Source: CAD feature listing. Evaluate the final solid. Frame: model axes, mm. A direction names the side the tool comes from. Coordinates: 2 decimals unless noted, no trailing zeros. Write each loop counter-clockwise with the first axis right and the second up, starting at its lowest first coordinate (ties: lowest second). Pieces come first, ordered by that corner, then holes. Notation, with made-up numbers: (-7.5, 42) - (50.5, 42) arc R7 cw to (50.5, 54) - close; hole circle Ø10 at (55, -12). An arc over 180 degrees is marked (long way). One line per item, written item: value.
from build123d import *

# Parameters (mm, degrees)
CROQUIS1_W              = 5.5
CROQUIS1_H              = 7
CROQUIS1_W_2            = 5
CROQUIS1_H_2            = 3
SALIENTE_EXTRUIR1_DEPTH = 20
CROQUIS2_W              = 5.5
CROQUIS2_H              = 7
CORTAR_EXTRUIR3_DEPTH   = 37.932370625
CROQUIS3_R              = 1.5
CORTAR_EXTRUIR4_DEPTH   = 33.015621187
REDONDEO1_R             = 3
CROQUIS4_R              = 1.5
CORTAR_EXTRUIR5_DEPTH   = 31.724582991
SALIENTE_EXTRUIR2_DEPTH = 20
CROQUIS9_R              = 2.75
CORTAR_EXTRUIR6_DEPTH   = 2.5


with BuildPart() as part:
    # Croquis1 → Saliente-Extruir1 (new body)
    with BuildSketch(Plane.XY):
        with Locations((-7.25, 3.5)):
            Rectangle(CROQUIS1_W, CROQUIS1_H)
        Polygon((0, -5), (0, -8), (-10, 0), (-4.5, 0), align=None)
        with Locations((2.5, -6.5)):
            Rectangle(CROQUIS1_W_2, CROQUIS1_H_2)
        with Locations((7.5, -6.5)):
            Rectangle(CROQUIS1_W_2, CROQUIS1_H_2)
        Polygon((14.5, 0), (20, 0), (10, -8), (10, -5), align=None)
        with Locations((17.25, 3.5)):
            Rectangle(CROQUIS1_W, CROQUIS1_H)
    extrude(amount=SALIENTE_EXTRUIR1_DEPTH)

    # Croquis2 → Cortar-Extruir3 (cut, through all)
    with BuildSketch(Plane.ZY.offset(10)):
        with Locations((15, 0)):
            Rectangle(CROQUIS2_W, CROQUIS2_H)
        with Locations((5, 0)):
            Rectangle(CROQUIS2_W, CROQUIS2_H)
    extrude(amount=-CORTAR_EXTRUIR3_DEPTH, mode=Mode.SUBTRACT)

    # Croquis3 → Cortar-Extruir4 (cut, through all)
    with BuildSketch(Plane(origin=(0, 7, 0), x_dir=(1, 0, 0), z_dir=(0, 1, 0))):
        with Locations(Location((-7.25, -5, 0), (0, 0, 180))):
            Circle(CROQUIS3_R)
        with Locations(Location((17.75, -5, 0), (0, 0, 180))):
            Circle(CROQUIS3_R)
        with Locations(Location((17.75, -15, 0), (0, 0, 180))):
            Circle(CROQUIS3_R)
        with Locations(Location((-7.25, -15, 0), (0, 0, 180))):
            Circle(CROQUIS3_R)
    extrude(amount=-CORTAR_EXTRUIR4_DEPTH, mode=Mode.SUBTRACT)

    # Redondeo1
    redondeo1_edges = [part.edges().sort_by_distance(p)[0] for p in [
        (20, 0, 18.875),
        (10, -8, 10),
        (0, -8, 10),
        (-10, 0, 18.875),
        (20, 0, 10),
        (20, 0, 1.125),
        (-10, 0, 10),
        (-10, 0, 1.125),
    ]]
    fillet(redondeo1_edges, radius=REDONDEO1_R)

    # Croquis4 → Cortar-Extruir5 (cut, through all)
    with BuildSketch(Plane(origin=(0, -5, 0), x_dir=(1, 0, 0), z_dir=(0, 1, 0))):
        with Locations(Location((5, -10, 0), (0, 0, 180))):
            Circle(CROQUIS4_R)
    extrude(amount=-CORTAR_EXTRUIR5_DEPTH, mode=Mode.SUBTRACT)

    # Croquis8 → Saliente-Extruir2 (add, through all)
    with BuildSketch(Plane(origin=(0, 0, 0), x_dir=(-1, 0, 0), z_dir=(0, 0, -1))):
        Polygon((-5, -5), (0, -5), (1.29685781, -3.559046878), (-5, -3.559046878), align=None)
        Polygon((-10, -5), (-5, -5), (-5, -3.559046878), (-11.29685781, -3.559046878), align=None)
    extrude(amount=-SALIENTE_EXTRUIR2_DEPTH)

    # Croquis9 → Cortar-Extruir6 (cut)
    with BuildSketch(Plane(origin=(0, -3.559046878, 0), x_dir=(1, 0, 0), z_dir=(0, 1, 0))):
        with Locations(Location((5, -10, 0), (0, 0, 180))):
            Circle(CROQUIS9_R)
    extrude(amount=-CORTAR_EXTRUIR6_DEPTH, mode=Mode.SUBTRACT)


solid = part.part
1) Section query C-C on z = 10. Output: boundary loops of the cut face in (x, y).
Values found:
outline: (-10, 1.44) arc R3 ccw to (-8.87, -0.9) - (-0.82, -7.34) arc R3 ccw to (1.05, -8) - (3.5, -8) - (3.5, -6.06) - (2.25, -6.06) - (2.25, -3.56) - (-1.3, -3.56) - (-4.5, 0) - (-4.5, 7) - (-10, 7) - close; (6.5, -8) - (8.95, -8) arc R3 ccw to (10.82, -7.34) - (18.87, -0.9) arc R3 ccw to (20, 1.44) - (20, 7) - (14.5, 7) - (14.5, 0) - (11.3, -3.56) - (7.75, -3.56) - (7.75, -6.06) - (6.5, -6.06) - close
2) Reachability of faces 4 (the flat face through (3.8, -6.059, 8.8)), 5 (the flat face through (2, -3.559, 10)), 6 (the flat face through (-7, 0, 2.25)), 7 (the cylindrical face through (-9.712, 0.159, 10.032)) from +Z, -Z, +X, -X, +Y, -Y: full face, straight path, thin tool, end or side. Return the list, or none.
Values found:
face 4: +Y
face 5: +Z, -Z, +Y
face 6: +X, -X
face 7: +Z, -Z, -X, -Y
3) Draft query along X for faces 1 (the cylindrical face through (19.25, 5.27, 5.07)), 2 (the flat face through (-6.1, 3.5, 6.2)), 3 (the cylindrical face through (19.7, 0.13, 10.03)). Return one class per face: released by +X, released by -X, zero draft, split by the parting line, or undercut.
Values found:
face 1: undercut
face 2: zero draft
face 3: released by +X
4) Contact query for flat-ended pins moving along their axis: P1, Ø3, axis at x = 16, z = 14.5, coming from the -Y side; P2, Ø3, axis at x = 17, z = 5.5, coming from the -Y side; P3, Ø2.5, axis at x = -7.25, z = 15, coming from the +Y side; P4, Ø2, axis at x = -2.5, z = 6, coming from the +Y side. Output: stop coordinate, or through.
Values found:
P1: y = -4.4
P2: y = -3.6
P3: through
P4: y = -3.5
5) Section query D-D on x = -7.25. Output: boundary loops of the cut face in (y, z), then the cut area to 3 significant figures.
Values found:
outline: (-2.2, 0) - (7, 0) - (7, 3.5) - (3.5, 3.5) - (3.5, 2.25) - (-2.2, 2.25) - close; (-2.2, 7.75) - (3.5, 7.75) - (3.5, 6.5) - (7, 6.5) - (7, 13.5) - (3.5, 13.5) - (3.5, 12.25) - (-2.2, 12.25) - close; (-2.2, 17.75) - (3.5, 17.75) - (3.5, 16.5) - (7, 16.5) - (7, 20) - (-2.2, 20) - close
area: 100 mm2
6) Section query A-A on z = 5. Output: boundary loops of the cut face in (x, y) (3 decimals), then the cut area to 3 significant figures.
Values found:
outline: (-10, 3.5) - (-8.75, 3.5) - (-8.75, 7) - (-10, 7) - close; (-5.75, 3.5) - (-4.5, 3.5) - (-4.5, 7) - (-5.75, 7) - close; (-5.625, -3.5) - (-0.822, -7.343) arc R3 ccw to (1.052, -8) - (8.948, -8) arc R3 ccw to (10.822, -7.343) - (15.625, -3.5) - (11.35, -3.5) - (11.297, -3.559) - (-1.297, -3.559) - (-1.35, -3.5) - close; (14.5, 3.5) - (16.25, 3.5) - (16.25, 7) - (14.5, 7) - close; (19.25, 3.5) - (20, 3.5) - (20, 7) - (19.25, 7) - close
area: 86.8 mm2
7) Material intervals for line 1 (Z direction, x = 14, y = -1.5); line 2 (Z direction, x = -7.25, y = 4.65); line 3 (X direction, y = 6, z = 8.75), sorted ascending.
Values found:
line 1: 0 to 2.25, 7.75 to 12.25, 17.75 to 20
line 2: 0 to 3.5, 6.5 to 13.5, 16.5 to 20
line 3: -10 to -4.5, 14.5 to 20
8) Section query B-B on y = 4.5. Output: boundary loops of the cut face in (x, z).
Values found:
outline: (-10, 0) - (-4.5, 0) - (-4.5, 20) - (-10, 20) - close; (14.5, 0) - (20, 0) - (20, 20) - (14.5, 20) - close; hole circle Ø3 at (-7.25, 5); hole circle Ø3 at (-7.25, 15); hole circle Ø3 at (17.75, 5); hole circle Ø3 at (17.75, 15)
